```python
from build123d import *

# Parameters (mm, degrees)
F0_W     = 101.125694
F0_H     = 101.125694
F0_R     = 31.418427
F1_DEPTH = 25.4
F0_R_2   = 23.299348
F2_DEPTH = 50.8


with BuildPart() as f1:
    # F0 (on Front) → F1 (new body)
    with BuildSketch(Plane.XZ):
        Rectangle(F0_W, F0_H)
        Circle(F0_R, mode=Mode.SUBTRACT)
    extrude(amount=F1_DEPTH)

    # F0 (on Front) → F2 (join)
    with BuildSketch(Plane.XZ):
        Circle(F0_R)
        Circle(F0_R_2, mode=Mode.SUBTRACT)
    extrude(amount=F2_DEPTH)


solid = f1.part
```
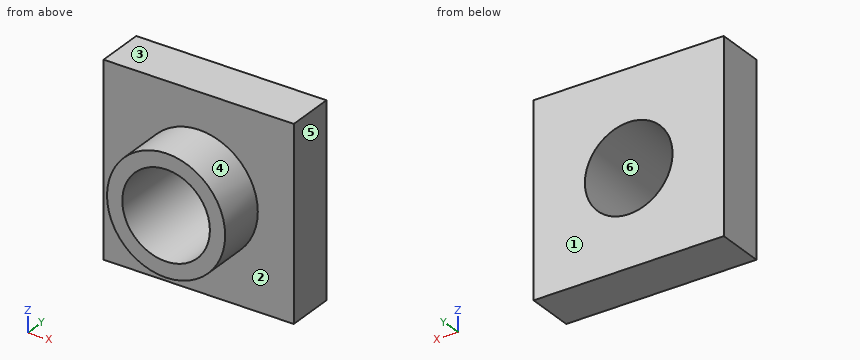
Model file for the job. Use its own axes, mm. Face numbers are marked on the shaded views. A direction names the side the tool comes from. Give positions to 0.01 mm unless a question says otherwise; leave off trailing zeros. Write each loop counter-clockwise with the first axis right and the second up, starting at its lowest first coordinate (ties: lowest second). Pieces come first, ordered by that corner, then holes. Notation, with made-up numbers: (81.25, 3.25) - (135.25, 3.25) arc R29 ccw to (135.25, 38.25) - close; hole circle Ø11 at (69.25, -3). An arc over 180 degrees is marked (long way). One line per question, with ' | ' between items. Start each with the question number.
(1) Wall check: line 1 along Z through (x, y) = (0, -14); line 2 along Z through (x, y) = (0, -29); line 3 along Y through (x, z) = (-22, 31). Give the ranges that are in metal, low to high. Write a range as from..to.
(2) Two-plate mould, pull along X, no slides. Class the marked faces 3, 4, 5 and 6: +X half, -X half, draft (parallel to the pull), parting line (faces both ways), or undercut.
(3) Slice it at C-C on y = -7. Write the cut outline in (x, z), plus the area to 3 significant figures.
(4) Slice it at B-B on x = 0. Write the cut outline in (y, z), plus the area to 3 significant figures.
(5) Slice it at A-A on z = 0. Write the cut outline in (x, y), plus the area to 3 significant figures.
(6) Pin check, flat tips, straight feed: P1, Ø5, axis at x = -38.5, z = -5, coming from the -Y side; P2, Ø1.5, axis at x = -38.5, y = -26.5, coming from the -Z side; P3, Ø8, axis at y = -30.5, z = 10.5, coming from the +X side; P4, Ø4, axis at y = -38.5, z = 28.5, coming from the +X side. Stop position of each tip, or through.
(7) 3-axis set-ups, long thin cutter, end or side, ignore diameter. For the marked faces 1 and 2: which of +Z, -Z, +X, -X, +Y, -Y reach the whole face in a straight line?
(8) Slice it at D-D on z = 26. Write the cut outline in (x, y).
Results below:
1) line 1: -50.56..-23.3, 23.3..50.56 | line 2: -31.42..-23.3, 23.3..31.42 | line 3: -25.4..0
2) face 3: draft | face 4: parting line | face 5: +X half | face 6: undercut
3) outline: (-50.56, -50.56) - (50.56, -50.56) - (50.56, 50.56) - (-50.56, 50.56) - close; hole circle Ø46.6 at (0, 0) | area: 8,520 mm^2
4) outline: (-50.8, -31.42) - (-25.4, -31.42) - (-25.4, -50.56) - (0, -50.56) - (0, -23.3) - (-50.8, -23.3) - close; (-50.8, 23.3) - (0, 23.3) - (0, 50.56) - (-25.4, 50.56) - (-25.4, 31.42) - (-50.8, 31.42) - close | area: 1,800 mm^2
5) outline: (-50.56, -25.4) - (-31.42, -25.4) - (-31.42, -50.8) - (-23.3, -50.8) - (-23.3, 0) - (-50.56, 0) - close; (23.3, -50.8) - (31.42, -50.8) - (31.42, -25.4) - (50.56, -25.4) - (50.56, 0) - (23.3, 0) - close | area: 1,800 mm^2
6) P1: y = -25.4 | P2: through | P3: x = 30.74 | P4: x = 16.88
7) face 1: +Z, -Z, +X, -X, +Y | face 2: -Y
8) outline: (-50.56, -25.4) - (-17.64, -25.4) - (-17.64, -50.8) - (17.64, -50.8) - (17.64, -25.4) - (50.56, -25.4) - (50.56, 0) - (-50.56, 0) - close
